from build123d import *

# Parameters (mm, degrees)
ESQUISSE1_W                 = 150
ESQUISSE1_H                 = 60
BOSS_EXTRU_1_DEPTH          = 37.5
ESQUISSE3_W                 = 140
ESQUISSE3_H                 = 52
ENL_V_MAT_EXTRU_2_DEPTH     = 70
ENL_V_MAT_VENTILATEUR_REACH = 159.5
ESQUISSE6_W                 = 30
ESQUISSE6_H                 = 30
ESQUISSE7_W                 = 2
ESQUISSE7_H                 = 4
BOSS_EXTRU_2_DEPTH          = 66
BOSS_EXTRU_3_DEPTH          = 30
ENL_V_MAT_ECRAN_REACH       = 105.108
ESQUISSE11_W                = 50
ESQUISSE11_H                = 34
ENL_V_MAT_MOLETTE_DEPTH     = 4
ESQUISSE15_W                = 2
ESQUISSE15_H                = 56
ENL_V_MAT_PAROI_DEPTH       = 147
BOSS_MOLETTE_DEPTH          = 2


with BuildPart() as part:
    # Esquisse1 → Boss.-Extru.1 (new, symmetric)
    with BuildSketch(Plane.XY):
        Rectangle(ESQUISSE1_W, ESQUISSE1_H)
    extrude(amount=BOSS_EXTRU_1_DEPTH, both=True)

    # Esquisse3 → Enlèv. mat.-Extru.2 (cut)
    with BuildSketch(Plane(origin=(0, 0, -37.5), x_dir=(-1, 0, 0), z_dir=(0, 0, -1))):
        Rectangle(ESQUISSE3_W, ESQUISSE3_H)
    extrude(amount=-ENL_V_MAT_EXTRU_2_DEPTH, mode=Mode.SUBTRACT)

    # Esquisse6 → Enlèv. mat.-Ventilateur (cut, up to next)
    with BuildSketch(Plane.ZY.offset(75), mode=Mode.PRIVATE) as enl_v_mat_ventilateur_sk1:
        with Locations((17.5, 10)):
            Rectangle(ESQUISSE6_W, ESQUISSE6_H)
    enl_v_mat_ventilateur_tool1 = extrude(enl_v_mat_ventilateur_sk1.sketch, amount=-ENL_V_MAT_VENTILATEUR_REACH, mode=Mode.PRIVATE) & part.part
    add(enl_v_mat_ventilateur_tool1.solids().sort_by_distance((-75, 10, 17.5))[0], mode=Mode.SUBTRACT)

    # Esquisse7 → Boss.-Extru.2 (add)
    with BuildSketch(Plane(origin=(0, 0, 32.5), x_dir=(-1, 0, 0), z_dir=(0, 0, -1))):
        with Locations((54, -24)):
            Rectangle(ESQUISSE7_W, ESQUISSE7_H)
    extrude(amount=BOSS_EXTRU_2_DEPTH)

    # Esquisse9 → Boss.-Extru.3 (add)
    with BuildSketch(Plane(origin=(0, 0, 32.5), x_dir=(-1, 0, 0), z_dir=(0, 0, -1))):
        Polygon((-70, 3.5), (53, 3.5), (53, 7.5), (55, 7.5), (55, 0), (-70, 0), align=None)
    extrude(amount=BOSS_EXTRU_3_DEPTH)

    # Esquisse11 → Enlèv. mat.-ecran (cut, up to next)
    with BuildSketch(Plane(origin=(0, 30, 0), x_dir=(1, 0, 0), z_dir=(0, 1, 0)), mode=Mode.PRIVATE) as enl_v_mat_ecran_sk1:
        with Locations((-18, -15.5)):
            Rectangle(ESQUISSE11_W, ESQUISSE11_H)
    enl_v_mat_ecran_tool1 = extrude(enl_v_mat_ecran_sk1.sketch, amount=-ENL_V_MAT_ECRAN_REACH, mode=Mode.PRIVATE) & part.part
    add(enl_v_mat_ecran_tool1.solids().sort_by_distance((-18, 30, 15.5))[0], mode=Mode.SUBTRACT)

    # Esquisse14 → Enlèv. mat.-molette (cut)
    with BuildSketch(Plane(origin=(0, 30, 0), x_dir=(1, 0, 0), z_dir=(0, 1, 0))):
        with BuildLine():
            Line((51, 17.5), (51, -29.5))
            ThreePointArc((51, -29.5), (48, -32.5), (45, -29.5))
            Line((45, -29.5), (45, 17.5))
            ThreePointArc((45, 17.5), (48, 20.5), (51, 17.5))
        make_face()
    extrude(amount=-ENL_V_MAT_MOLETTE_DEPTH, mode=Mode.SUBTRACT)

    # Esquisse15 → Enlèv. mat.-paroi (cut)
    with BuildSketch(Plane.ZY.offset(75)):
        with Locations((-34.5, 0)):
            Rectangle(ESQUISSE15_W, ESQUISSE15_H)
    extrude(amount=-ENL_V_MAT_PAROI_DEPTH, mode=Mode.SUBTRACT)

    # Esquisse16 → Boss.-molette (add)
    with BuildSketch(Plane(origin=(0, 3.5, 0), x_dir=(1, 0, 0), z_dir=(0, 1, 0))):
        Polygon((64, -32.5), (64, -12.5), (32, -12.5), (32, -32.5), (30, -32.5), (30, -10.5), (66, -10.5), (66, -32.5), align=None)
    extrude(amount=BOSS_MOLETTE_DEPTH)


solid = part.part
Could you check a few things on this model? Use its own coordinates, in mm. A direction names the side the tool comes from. Give positions to 0.01 mm unless a question says otherwise; leave off trailing zeros. Order: outer loops, then holes, each group sorted by start corner. A loop starts at its lowest first (then second) coordinate and runs counter-clockwise, first axis right, second up. Notation, with made-up numbers: (12, 63) - (53, 63) arc R26 ccw to (53, 95) - close; hole circle Ø11 at (18.25, -11). An arc over 180 degrees is marked (long way). Return JSON: item names as keys, results as strings. Group by question number.
Q1. Suppose I cut it at C-C, the plane z = -8. Please give me the cut outline in (x, y).
Q2. Please list where these lines run through material, in increasing order: line 1 along Y through (x, z) = (23, 28); line 2 along Y through (x, z) = (31, 29); line 3 along X through (y, z) = (-25, 12). Write a range as [from, to].
Q3. Thinking about a two-plate mould opening in Z: for faces 1 (the face through (-75, 0, 1)), 2 (the face through (7, 28, 16)), 3 (the face through (-1, 0, 37.5)), which applies, pulls with the +Z half, pulls with the -Z half, needs draft (parallel to the pull), parting line crosses it, or undercut?
Q4. Suppose I cut it at D-D, the plane y = 13. Please give me the cut outline in (x, z).
Q5. Will these pins go through, and if not, where does the flat tip stop? pin 1 Ø0.6 at (y, z) = (4.5, 21.5) entering from -X; pin 2 Ø8 at (x, y) = (16.5, 17) entering from -Z; pin 3 Ø4 at (x, y) = (17, 0) entering from -Z.
Q6. Suppose I cut it at A-A, the plane z = 6.5. State how many separate pieces and enclosed holes the cut face has, and give its area (3 significant figures).
Q7. Suppose I cut it at B-B, the plane y = -15. Please give me the cut outline in (x, z), and give its area (3 significant figures).
Q8. Which directions (+Z, -Z, +X, -X, +Y, -Y) give clear straight access to the entire face, cutting with the end or side of a thin tool? Please do faces 4 (the face through (-62, -26, -1)), 5 (the face through (48, 3.5, 23)), 6 (the face through (-24, 27, -35.5)), 7 (the face through (45, 28, 6)), 8 (the face through (7, 0, 18)).
Resolved:
{
 "1": {"outline": "(-75, -30) - (75, -30) - (75, 30) - (51, 30) - (51, 26) - (70, 26) - (70, -26) - (-53, -26) - (-53, -22) - (-55, -22) - (-55, -26) - (-70, -26) - (-70, 26) - (45, 26) - (45, 30) - (-75, 30) - close"},
 "2": {"line 1": "y = [-30, -26], [0, 3.5], [26, 30]", "line 2": "y = [-30, -26], [0, 5.5], [26, 30]", "line 3": "x = [-75, -70], [-55, -53], [70, 75]"},
 "3": {"face 1": "needs draft", "face 2": "undercut", "face 3": "pulls with the +Z half"},
 "4": {"outline": "(-75, -37.5) - (-70, -37.5) - (-70, -35.5) - (-75, -35.5) - close; (-75, -33.5) - (-70, -33.5) - (-70, 2.5) - (-75, 2.5) - close; (-75, 32.5) - (70, 32.5) - (70, -33.5) - (72, -33.5) - (72, -35.5) - (70, -35.5) - (70, -37.5) - (75, -37.5) - (75, 37.5) - (-75, 37.5) - close"},
 "5": {"pin 1": "stops at x = -55", "pin 2": "stops at z = 32.5", "pin 3": "stops at z = 2.5"},
 "6": {"separate pieces": "3", "enclosed holes": "0", "area": "1,800 mm2"},
 "7": {"outline": "(-75, -37.5) - (-70, -37.5) - (-70, -35.5) - (-75, -35.5) - close; (-75, -33.5) - (-70, -33.5) - (-70, 32.5) - (70, 32.5) - (70, -33.5) - (72, -33.5) - (72, -35.5) - (70, -35.5) - (70, -37.5) - (75, -37.5) - (75, 37.5) - (-75, 37.5) - close", "area": "1,440 mm2"},
 "8": {"face 4": "-Z", "face 5": "none", "face 6": "-X", "face 7": "+Y", "face 8": "-Z, -X"}
}
